Geometry check sheet. Reference: the model listing, model coordinates, mm. Round coordinates to 2 decimals unless told otherwise and drop trailing zeros. Order: outer loops, then holes, each group sorted by start corner. A loop starts at its lowest first (then second) coordinate and runs counter-clockwise, first axis right, second up. Notation, with made-up numbers: (-11.75, 20.25) -> (7.25, 20.25) arc R9 cw to (7.25, 30.25) -> close; hole circle Ø5 at (57, 58). An arc over 180 degrees is marked (long way). Answer as a JSON object with one key per item and string values. Group by question number.
Autodesk Inventor part; units mm, degrees
ref_plane "YZ Plane" through (0, 0, 0) normal (1, 0, 0) x (0, 1, 0)
ref_plane "XZ Plane" through (0, 0, 0) normal (0, 1, 0) x (-1, 0, 0)
ref_plane "XY Plane" through (0, 0, 0) normal (0, 0, 1) x (1, 0, 0)
sketch "Sketch1" plane through (0, 0, 0) normal (0, 1, 0) x (-1, 0, 0)
  circle A0 centre (0, 0) radius 45
  dimension "d0" = 90
extrude "Extrusion1" add sketch "Sketch1" along normal blind 50
sketch "Sketch2" plane through (0, 0, 0) normal (1, 0, 0) x (0, 1, 0)
  line L0 (50, -45) -> (50, 45)
  line L1 (50, 45) -> (50.7071, 45.7071)
  line L2 (50.7071, 45.7071) -> (90, 45) construction
  line L3 (90, 45) -> (126, 40) construction
  line L4 (126, 40) -> (125, 0) construction
  spline S0 degree 3 poles (50.7071, 45.7071) (90, 45) (126, 40) (125, 0) knots 1 1 1 1 2 2 2 2
  line L5 (125, 0) -> (50, 0)
  line L6 (50, 0) -> (50, 45)
  point P0 (0, 0)
  dimension "d3" = 1
  dimension "d4" = 135
  dimension "d5" = 40
  dimension "d6" = 76
  dimension "d7" = 75
  dimension "d8" = 40
  dimension "d9" = 45
revolve "Revolution1" add sketch "Sketch2" angle 360 about axis through (0, 125, 0) along (0, -1, 0)
fillet "Fillet1" radius 2.3 2 edges at (31.8198, 50, -31.8198) (-31.8198, 50, 31.8198)
sketch "Sketch3" plane through (0, 0, 0) normal (0, -1, 0) x (1, 0, 0)
  line L0 (34.641, 0) -> (-17.3205, 30) construction
  line L1 (-17.3205, 30) -> (-17.3205, -30) construction
  line L2 (-17.3205, -30) -> (34.641, 0) construction
  circle A0 centre (0, 0) radius 34.641 construction
  circle A1 centre (-17.3205, 30) radius 6.25
  circle A2 centre (34.641, 0) radius 6.25
  circle A3 centre (-17.3205, -30) radius 6.25
  point P0 (-17.3205, 0)
  dimension "d12" = 60
  dimension "d13" = 12.5
extrude "Extrusion2" add sketch "Sketch3" along normal blind 5
sketch "Sketch4" plane through (-17.3205, -5, 30) normal (0, -1, 0) x (1, 0, 0)
  circle A0 centre (0, 0) radius 6.25
  circle A1 centre (0, 0) radius 1.5
  point P0 (17.3205, -30)
  dimension "d16" = 3
extrude "Extrusion3" add sketch "Sketch4" along normal blind 15 contours A1
chamfer "Chamfer1" distance 0.5 angle 45 1 edges at (-18.8205, -20, 30)
thread "Thread1"
pattern_circular "Circular Pattern1" count 3 over 360 about axis through (0, 0, 0) along (0, 1, 0) of "Extrusion3", "Chamfer1"
properties part number "Circulina" material "Steel, Mild, Welded"
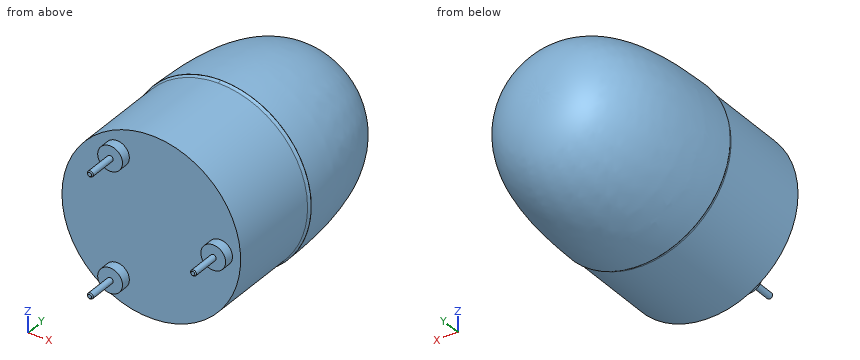
Item 1: Depth check by flat-ended pin: pin 1 Ø10 at (x, y) = (6, 34.5) entering from -Z; pin 2 Ø3 at (y, z) = (72.5, 4) entering from -X; pin 3 Ø2 at (x, y) = (3.5, 104.5) entering from -Z. Enter the tip coordinate at first touch or a pass-through.
Item 2: Thickness scan on L1, parallel to Y at x = -16, z = -34; L2, parallel to Y at x = 9.5, z = -34; L3, parallel to X at y = 18, z = 38.5. Record the ranges inside material, lowest first.
Item 3: Sectioned sample at A-A, the plane y = 33. Enter the section's corners in (x, z), then the cut area to 3 significant figures.
Result:
{
 "1": {"pin 1": "stops at z = -44.99", "pin 2": "stops at x = -44.63", "pin 3": "stops at z = -37.18"},
 "2": {"L1": "y = -5 to 102.99", "L2": "y = 0 to 107.34", "L3": "x = -23.3 to 23.3"},
 "3": {"outline": "circle Ø90 at (0, 0)", "area": "6,360 mm2"}
}
